```python
from build123d import *

# Parameters (mm, degrees)
BOSS_EXTRUDE1_DEPTH = 50
SCALE1_SCALE        = 0.04


with BuildPart() as part:
    # Sketch1 → Boss-Extrude1 (new body)
    with BuildSketch(Plane.XY):
        Polygon((0, 6238.869420035), (0, 5457.819420035), (50.8, 5457.819420035), (50.8, 4937.119420035), (0, 4937.119420035), (0, 4416.419420035), (50.8, 4416.419420035), (50.8, 3895.719420035), (0, 3895.719420035), (0, 3375.019420035), (50.8, 3375.019420035), (50.8, 2854.319420035), (0, 2854.319420035), (0, 2333.619420035), (50.8, 2333.619420035), (50.8, 1812.919420035), (0, 1812.919420035), (0, 1292.219420035), (50.8, 1292.219420035), (50.8, 771.519420035), (0, 771.519420035), (0, 250.819420035), (0, -9.530579965), (488.95, -9.530579965), (488.95, -60.330579965), (1009.65, -60.330579965), (1009.65, -9.530579965), (1530.35, -9.530579965), (1530.35, -60.330579965), (2051.05, -60.330579965), (2051.05, -9.530579965), (2540, -9.530579965), (2540, 771.519420035), (2489.2, 771.519420035), (2489.2, 1292.219420035), (2540, 1292.219420035), (2540, 1812.919420035), (2489.2, 1812.919420035), (2489.2, 2333.619420035), (2540, 2333.619420035), (2540, 2854.319420035), (2489.2, 2854.319420035), (2489.2, 3375.019420035), (2540, 3375.019420035), (2540, 3895.719420035), (2489.2, 3895.719420035), (2489.2, 4416.419420035), (2540, 4416.419420035), (2540, 4937.119420035), (2489.2, 4937.119420035), (2489.2, 5457.819420035), (2540, 5457.819420035), (2540, 5978.519420035), (2540, 6238.869420035), (2051.05, 6238.869420035), (2051.05, 6289.669420035), (1530.35, 6289.669420035), (1530.35, 6238.869420035), (1009.65, 6238.869420035), (1009.65, 6289.669420035), (488.95, 6289.669420035), (488.95, 6238.869420035), align=None)
    extrude(amount=BOSS_EXTRUDE1_DEPTH)


with BuildPart() as part_1:
    # Scale1: scaled about (1270, 3114.669420035, 25)
    add(part.part.scale(SCALE1_SCALE).moved(Location((1219.2, 2990.082643234, 24))))


solid = part_1.part
```
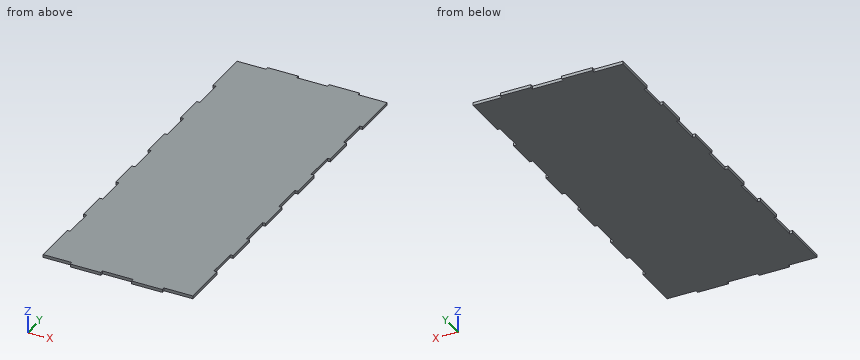
Geometry: final body of the model. Coordinates: model frame, mm. Coordinates: 2 decimals unless noted, no trailing zeros. Order: outer loops, then holes, each group sorted by start corner. A loop starts at its lowest first (then second) coordinate and runs counter-clockwise, first axis right, second up.
Item 1: Material intervals for line 1 along X through (y, z) = (3028, 24.5); line 2 along Y through (x, z) = (1229, 25.2), sorted ascending.
Answer:
line 1: x = 1221.23 to 1318.77
line 2: y = 2989.7 to 3239.64
Item 2: Contact query for flat-ended pins moving along their axis: P1, Ø1, axis at x = 1319.5, z = 24.5, coming from the +Y side; P2, Ø1, axis at y = 3034, z = 24.5, coming from the +X side; P3, Ø0.6, axis at y = 2989, z = 25.5, coming from the +X side. Output: stop coordinate, or through.
Answer:
P1: stops at y = 3239.64
P2: stops at x = 1318.77
P3: stops at x = 1301.24
Item 3: Section query A-A (x = 1309.5). Output: boundary loops of the cut face in (y, z).
Answer:
outline: (2989.7, 24) - (3239.64, 24) - (3239.64, 26) - (2989.7, 26) - close
